CAD build for the part. Positions are in the model's coordinates, mm. Face numbers are marked on the shaded views. A direction names the side the tool comes from. Give positions to 0.01 mm unless a question says otherwise; leave off trailing zeros. Loops run counter-clockwise (first coordinate to the right, second up) from the corner with the lowest first, then second, coordinate; pieces in that order, holes last. Notation, with made-up numbers: M 78,-30 L 136,-30 A20 ccw 136,-7 Z; hole C 19.5,41 d6. An arc over 180 degrees is marked long. Answer as CSV lines item,"result".
```python
from build123d import *

# Parameters (mm, degrees)
SKETCH1_W            = 35.2
SKETCH1_H            = 49.5
BOSS_EXTRUDE1_DEPTH  = 2.3
SKETCH2_W            = 2.3
SKETCH2_H            = 49.5
BOSS_EXTRUDE2_DEPTH  = 4.8
SKETCH3_W            = 83.5
SKETCH3_H            = 49.5
BOSS_EXTRUDE3_DEPTH  = 2.3
CUT_EXTRUDE1_DEPTH   = 50.436676668
BOSS_EXTRUDE10_DEPTH = 69.5
SKETCH7_W            = 7
SKETCH7_H            = 7
SKETCH7_R            = 1.75
BOSS_EXTRUDE7_DEPTH  = 2.3
CHAMFER1_SIZE        = 0.5
SKETCH12_W           = 7
SKETCH12_H           = 2.3
BOSS_EXTRUDE11_DEPTH = 8.8
SKETCH13_W           = 2.3
SKETCH13_H           = 2.3
SKETCH13_W_2         = 1
BOSS_EXTRUDE12_DEPTH = 36
SKETCH14_R           = 1
SKETCH14_R_2         = 2
CUT_EXTRUDE3_DEPTH   = 135.201723163
CUT_EXTRUDE4_REACH   = 164.416
SKETCH18_R           = 4
SKETCH18_W           = 9
SKETCH18_H           = 15
CHAMFER2_SIZE        = 1


with BuildPart() as part:
    # Sketch1 → Boss-Extrude1 (new body)
    with BuildSketch(Plane.XY):
        Rectangle(SKETCH1_W, SKETCH1_H)
    extrude(amount=BOSS_EXTRUDE1_DEPTH)

    # Sketch2 → Boss-Extrude2 (add)
    with BuildSketch(Plane.XY.offset(2.3)):
        Rectangle(SKETCH2_W, SKETCH2_H)
    extrude(amount=BOSS_EXTRUDE2_DEPTH)

    # Sketch3 → Boss-Extrude3 (add)
    with BuildSketch(Plane.XY.offset(7.1)):
        Rectangle(SKETCH3_W, SKETCH3_H)
    extrude(amount=BOSS_EXTRUDE3_DEPTH)

    # Sketch4 → Cut-Extrude1 (cut, through all)
    with BuildSketch(Plane.XY.offset(9.4)):
        with BuildLine():
            Line((-34.25, 2.45), (-40.75, 2.45))
            Line((-40.75, 2.45), (-40.75, -2.45))
            Line((-40.75, -2.45), (-34.25, -2.45))
            ThreePointArc((-34.25, -2.45), (-36.7, 0), (-34.25, 2.45))
        make_face()
        with BuildLine():
            ThreePointArc((-31.8, 0), (-32.517588386, 1.732411614), (-34.25, 2.45))
            Line((-34.25, 2.45), (-34.25, -2.45))
            ThreePointArc((-34.25, -2.45), (-32.517588386, -1.732411614), (-31.8, 0))
        make_face()
        with BuildLine():
            Line((-34.25, -2.45), (-34.25, 2.45))
            ThreePointArc((-34.25, 2.45), (-36.7, 0), (-34.25, -2.45))
        make_face()
        with BuildLine():
            ThreePointArc((34.25, 2.45), (31.8, 0), (34.25, -2.45))
            Line((34.25, -2.45), (34.25, 2.45))
        make_face()
        with BuildLine():
            Line((34.25, 2.45), (34.25, -2.45))
            ThreePointArc((34.25, -2.45), (35.982411614, -1.732411614), (36.7, 0))
            ThreePointArc((36.7, 0), (35.982411614, 1.732411614), (34.25, 2.45))
        make_face()
        with BuildLine():
            Line((34.25, -2.45), (40.75, -2.45))
            Line((40.75, -2.45), (40.75, 2.45))
            Line((40.75, 2.45), (34.25, 2.45))
            ThreePointArc((34.25, 2.45), (35.982411614, 1.732411614), (36.7, 0))
            ThreePointArc((36.7, 0), (35.982411614, -1.732411614), (34.25, -2.45))
        make_face()
    extrude(amount=-CUT_EXTRUDE1_DEPTH, mode=Mode.SUBTRACT)

    # Sketch10 → Boss-Extrude10 (add)
    with BuildSketch(Plane.XZ.offset(24.75)):
        Polygon((-41.75, 7.1), (-41.75, 9.4), (-57.5, 9.4), (-57.5, -105.6), (57.5, -105.6), (57.5, 9.4), (41.75, 9.4), (41.75, 7.1), (55.2, 7.1), (55.2, -103.3), (-55.2, -103.3), (-55.2, 7.1), align=None)
    extrude(amount=-BOSS_EXTRUDE10_DEPTH)

    # Sketch7 → Boss-Extrude7 (add)
    with BuildSketch(Plane.XZ.offset(24.75)):
        with Locations((-24.2, 3.6)):
            Rectangle(SKETCH7_W, SKETCH7_H)
        with Locations(Location((-24.2, 3.6, 0), (0, 0, 270))):
            Circle(SKETCH7_R, mode=Mode.SUBTRACT)
        with Locations((24.2, 3.6)):
            Rectangle(SKETCH7_W, SKETCH7_H)
        with Locations(Location((24.2, 3.6, 0), (0, 0, 90))):
            Circle(SKETCH7_R, mode=Mode.SUBTRACT)
        with Locations((24.2, -99.8)):
            Rectangle(SKETCH7_W, SKETCH7_H)
        with Locations(Location((24.2, -99.8, 0), (0, 0, 270))):
            Circle(SKETCH7_R, mode=Mode.SUBTRACT)
        with Locations((-24.2, -99.8)):
            Rectangle(SKETCH7_W, SKETCH7_H)
        with Locations(Location((-24.2, -99.8, 0), (0, 0, 90))):
            Circle(SKETCH7_R, mode=Mode.SUBTRACT)
    extrude(amount=-BOSS_EXTRUDE7_DEPTH)

    # Chamfer1
    chamfer1_edges = [part.edges().sort_by_distance(p)[0] for p in [
        (-27.7, -23.6, 7.1),
        (-20.7, -23.6, 7.1),
        (27.7, -23.6, 7.1),
        (20.7, -23.6, 7.1),
        (27.7, -23.6, -103.3),
        (20.7, -23.6, -103.3),
        (-27.7, -23.6, -103.3),
        (-20.7, -23.6, -103.3),
    ]]
    chamfer(chamfer1_edges, length=CHAMFER1_SIZE)

    # Sketch12 → Boss-Extrude11 (add)
    with BuildSketch(Plane.XY.offset(-103.3)):
        with Locations((51.7, -23.6)):
            Rectangle(SKETCH12_W, SKETCH12_H)
        with Locations((-51.7, -23.6)):
            Rectangle(SKETCH12_W, SKETCH12_H)
    extrude(amount=BOSS_EXTRUDE11_DEPTH)

    # Sketch13 → Boss-Extrude12 (add)
    with BuildSketch(Plane(origin=(0, -22.45, 0), x_dir=(1, 0, 0), z_dir=(0, 1, 0))):
        with Locations((54.05, 95.65)):
            Rectangle(SKETCH13_W, SKETCH13_H)
        with Locations((-54.7, 95.65)):
            Rectangle(SKETCH13_W_2, SKETCH13_H)
    extrude(amount=BOSS_EXTRUDE12_DEPTH)

    # Sketch14 → Cut-Extrude3 (cut, through all)
    with BuildSketch(Plane.XY.offset(-103.3)):
        with Locations((46.7, -4.7)):
            Circle(SKETCH14_R)
        with Locations((38.2, -4.7)):
            Circle(SKETCH14_R)
        with Locations((29.7, -4.7)):
            Circle(SKETCH14_R)
        with Locations((21.2, -4.7)):
            Circle(SKETCH14_R)
        with Locations((3.8, -4.7)):
            Circle(SKETCH14_R_2)
    extrude(amount=-CUT_EXTRUDE3_DEPTH, mode=Mode.SUBTRACT)

    # Sketch18 → Cut-Extrude4 (cut, up to next)
    with BuildSketch(Plane.ZY.offset(57.5), mode=Mode.PRIVATE) as cut_extrude4_sk1:
        with Locations((-89.6, -20.71)):
            Circle(SKETCH18_R)
    cut_extrude4_tool1 = extrude(cut_extrude4_sk1.sketch, amount=-CUT_EXTRUDE4_REACH, mode=Mode.PRIVATE) & part.part
    # Sketch18 → Cut-Extrude4 (cut, up to next)
    with BuildSketch(Plane.ZY.offset(57.5), mode=Mode.PRIVATE) as cut_extrude4_sk2:
        with Locations((-81.6, -20.71)):
            Circle(SKETCH18_R)
    cut_extrude4_tool2 = extrude(cut_extrude4_sk2.sketch, amount=-CUT_EXTRUDE4_REACH, mode=Mode.PRIVATE) & part.part
    # Sketch18 → Cut-Extrude4 (cut, up to next)
    with BuildSketch(Plane.ZY.offset(57.5), mode=Mode.PRIVATE) as cut_extrude4_sk3:
        with Locations((-85.6, -17.25)):
            Rectangle(SKETCH18_W, SKETCH18_H)
    cut_extrude4_tool3 = extrude(cut_extrude4_sk3.sketch, amount=-CUT_EXTRUDE4_REACH, mode=Mode.PRIVATE) & part.part
    add(cut_extrude4_tool1.solids().sort_by_distance((-57.5, -20.71, -89.6))[0], mode=Mode.SUBTRACT)
    add(cut_extrude4_tool2.solids().sort_by_distance((-57.5, -20.71, -81.6))[0], mode=Mode.SUBTRACT)
    add(cut_extrude4_tool3.solids().sort_by_distance((-57.5, -17.25, -85.6))[0], mode=Mode.SUBTRACT)

    # Chamfer2
    chamfer2_edges = [part.edges().sort_by_distance(p)[0] for p in [
        (-56.35, -9.75, -81.1),
        (-56.35, -9.75, -90.1),
    ]]
    chamfer(chamfer2_edges, length=CHAMFER2_SIZE)


solid = part.part
```
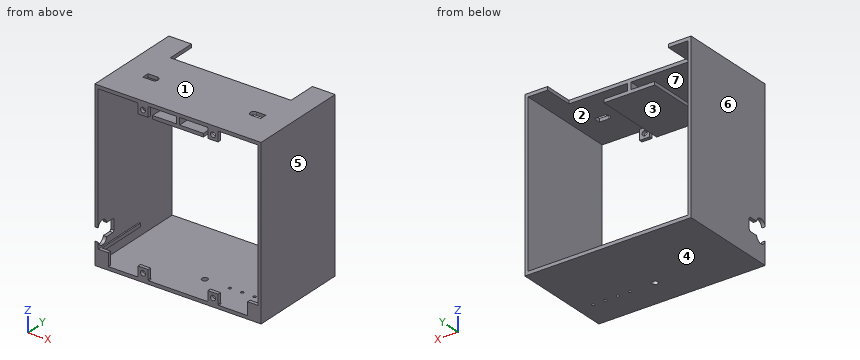
Q1. Cut at D-D (y = 15). Write the cut outline in (x, z), and give its area (3 significant figures).
Solution:
outline,"M -57.5,-105.6 L 57.5,-105.6 L 57.5,9.4 L -57.5,9.4 Z; hole M -55.2,-103.3 L 55.2,-103.3 L 55.2,7.1 L 1.15,7.1 L 1.15,2.3 L 17.6,2.3 L 17.6,0 L -17.6,0 L -17.6,2.3 L -1.15,2.3 L -1.15,7.1 L -55.2,7.1 Z"
area,"1,130 mm²"
Q2. Mould opens along X. For the marked faces 4, 5, 6 and 7 say: released by +X, released by -X, zero draft, split by the parting line, or undercut.
Solution:
face 4,"zero draft"
face 5,"released by +X"
face 6,"released by -X"
face 7,"undercut"
Q3. Cut at C-C (x = 3.8). Write the cut outline in (y, z), and give its area (3 significant figures).
Solution:
outline,"M -24.75,-105.6 L -6.7,-105.6 L -6.7,-103.3 L -24.75,-103.3 Z; M -24.75,0 L 24.75,0 L 24.75,2.3 L -24.75,2.3 Z; M -24.75,7.1 L 24.75,7.1 L 24.75,9.4 L -24.75,9.4 Z; M -2.7,-105.6 L 44.75,-105.6 L 44.75,-103.3 L -2.7,-103.3 Z"
area,"378 mm²"
Q4. Wall check: line 1 (Z direction, x = -15.5, y = -14); line 2 (X direction, y = -23.5, z = -99.8); line 3 (X direction, y = -15.5, z = -19). Give the ranges that are in metal, low to high. Write a range as [from, to].
Solution:
line 1,"z = [-105.6, -103.3], [0, 2.3], [7.1, 9.4]"
line 2,"x = [-57.5, -48.2], [-27.7, -25.95], [-22.45, -20.7], [20.7, 22.45], [25.95, 27.7], [48.2, 57.5]"
line 3,"x = [-57.5, -55.2], [55.2, 57.5]"
Q5. Cut at B-B (z = -35). Write the cut outline in (x, y), and give its area (3 significant figures).
Solution:
outline,"M -57.5,-24.75 L -55.2,-24.75 L -55.2,44.75 L -57.5,44.75 Z; M 55.2,-24.75 L 57.5,-24.75 L 57.5,44.75 L 55.2,44.75 Z"
area,"320 mm²"
Q6. Which spindle directions (+Z, -Z, +X, -X, +Y, -Y) get a long thin tool onto all of the face, cutting with end or side? Do the marked faces 1, 2 and 3. Say none if no direction does.
Solution:
face 1,"+Z, +X, -X, +Y, -Y"
face 2,"+Y"
face 3,"+Y, -Y"
Q7. Pin check, flat tips, straight feed: P1, Ø1.8, axis at x = 29.7, y = -4.7, coming from the -Z side; P2, Ø1.1, axis at x = -56.5, z = -86.5, coming from the -Y side; P3, Ø5.5, axis at x = 23, z = 4, coming from the +Y side. Stop position of each tip, or through.
Solution:
P1,"stops at z = 7.1"
P2,"stops at y = -9.75"
P3,"stops at y = -22.45"
Q8. Cut at A-A (x = -9). Write the cut outline in (y, z).
Solution:
outline,"M -24.75,-105.6 L 44.75,-105.6 L 44.75,-103.3 L -24.75,-103.3 Z; M -24.75,0 L 24.75,0 L 24.75,2.3 L -24.75,2.3 Z; M -24.75,7.1 L 24.75,7.1 L 24.75,9.4 L -24.75,9.4 Z"
